Answer from the drawing. Dimensions are ordinates in mm from the lowest x, y and z of the part. Round coordinates to 2 decimals unless told otherwise and drop trailing zeros. Order: outer loops, then holes, each group sorted by start corner. A loop starts at its lowest first (then second) coordinate and runs counter-clockwise, first axis right, second up. Notation, with made-up numbers: (21.25, 39.25) -> (31.25, 39.25) arc R9 cw to (31.25, 49.25) -> close; hole circle Ø3 at (31.5, 44.5). An arc over 180 degrees is marked (long way). Use a Markdown table: item, result. Add a question column.
Item 1: A cutting plane is placed at D-D, the plane x = 49.5. Determine the outline of the cut face in (y, z), plus the area to 3 significant figures.
Item 2: A cutting plane is placed at C-C, the plane z = 14. Determine the outline of the cut face in (x, y), plus the area to 3 significant figures.
Item 3: Flat-ended cylindrical pins translate along their axes: P1, Ø1, axis at x = 14.5, z = 3.5, coming from the +Y side; P2, Ø6, axis at x = 33.5, z = 24, coming from the +Y side; P3, Ø1, axis at y = 3, z = 7, coming from the +X side (3 decimals); P4, Ø2, axis at x = 18, z = 13.5, coming from the -Y side. Find the tip coordinate at first contact, or state that the pin passes through.
Item 4: Find the intervals of material crossed by L1, parallel to Z at x = 37.5, y = 15.25; L2, parallel to X at y = 15.25, z = 13.5; L3, parallel to Z at x = 54, y = 19.25, in increasing order. Write a range as [from, to].
Item 5: A cutting plane is placed at B-B, the plane x = 39.5. Determine the outline of the cut face in (y, z), plus the area to 3 significant figures.
Item 6: A cutting plane is placed at A-A, the plane y = 7. Determine the outline of the cut face in (x, z).
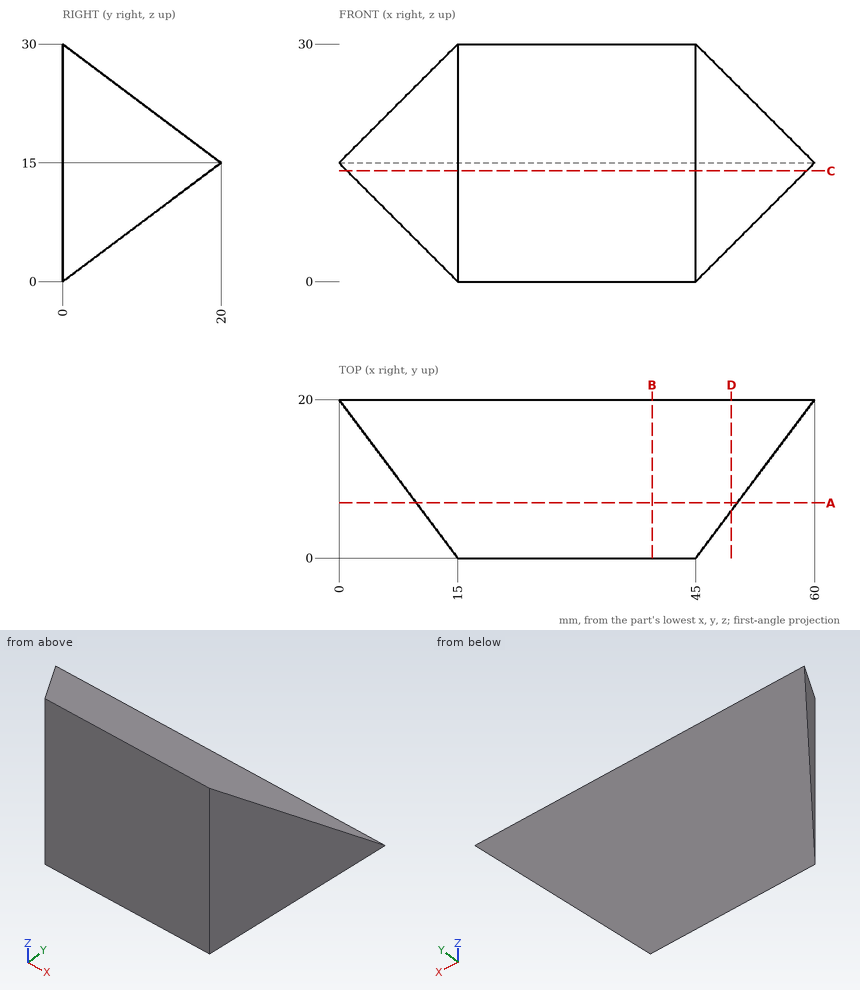
Reported:
| question | item | result |
|---|---|---|
| 1 | outline | (6, 4.5) -> (20, 15) -> (6, 25.5) -> close |
| 1 | area | 147 mm² |
| 2 | outline | (1, 18.67) -> (15, 0) -> (45, 0) -> (59, 18.67) -> close |
| 2 | area | 821 mm² |
| 3 | P1 | y = 5.33 |
| 3 | P2 | y = 12 |
| 3 | P3 | x = 47.625 |
| 3 | P4 | y = 0 |
| 4 | L1 | [11.44, 18.56] |
| 4 | L2 | [3.56, 56.44] |
| 4 | L3 | [14.44, 15.56] |
| 5 | outline | (0, 0) -> (20, 15) -> (0, 30) -> close |
| 5 | area | 300 mm² |
| 6 | outline | (9.75, 5.25) -> (50.25, 5.25) -> (50.25, 24.75) -> (9.75, 24.75) -> close |
